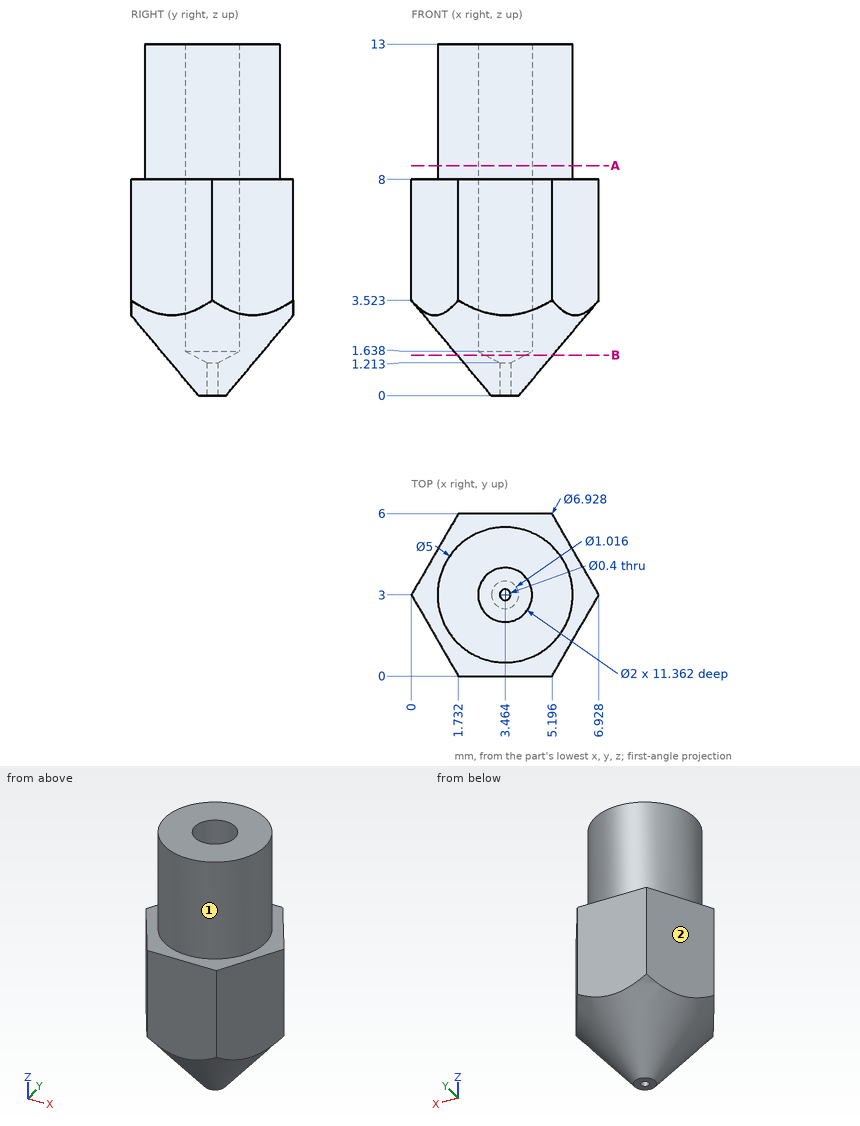
Job drawing, mm, ordinate dimensions from the low corner. One solid piece. A direction names the side the tool comes from. Give positions to 0.01 mm unless a question says otherwise; leave off trailing zeros. Loops run counter-clockwise (first coordinate to the right, second up) from the corner with the lowest first, then second, coordinate; pieces in that order, holes last. Notation, with made-up numbers: M -19,-20 L -9,-20 A28 ccw -9,7 Z; hole C 36,-22 d9. An arc over 180 degrees is marked long. Use one line per item in the form item = value.
Item 1: Flat gauge pins, fed straight in: pin 1 Ø1 at (x, y) = (4.5, 5) entering from -Z; pin 2 Ø1.8 at (x, y) = (3.46, 3) entering from +Z; pin 3 Ø2 at (x, y) = (2.5, 2) entering from -Z; pin 4 Ø3 at (y, z) = (1.5, 2) entering from +X. Where does each tip first touch, or does it go through?
Filled in:
pin_1 = 1.48
pin_2 = 1.59
pin_3 = 0
pin_4 = 6.59
Item 2: Slice it at B-B on z = 1.5. List the corners of the cut face in (x, y).
Filled in:
outline = C 3.46,3 d3.53; hole C 3.46,3 d1.48
Item 3: Which spindle directions (+Z, -Z, +X, -X, +Y, -Y) get a long thin tool onto all of the face, cutting with end or side? Do the marked faces 1 and 2. Say none if no direction does.
Filled in:
face_1 = +Z
face_2 = +Z, -Z, -X, +Y
Item 4: Drill centre lines: L1, parallel to X at y = 3.25, z = 8.5; L2, parallel to X at y = 2.5, z = 8.25 (1 decimal); L3, parallel to Y at x = 4.25, z = 10.25 (1 decimal). Where is each one in solid material? Low to high.
Filled in:
L1 = 0.98 to 2.5, 4.43 to 5.95
L2 = 1 to 2.6, 4.3 to 5.9
L3 = 0.6 to 2.4, 3.6 to 5.4
Item 5: Slice it at A-A on z = 8.5. List the corners of the cut face in (x, y), and give its area (3 significant figures).
Filled in:
outline = C 3.46,3 d5; hole C 3.46,3 d2
area = 16.5 mm^2
